Source: three-view drawing plus pictorial views. Frame: mm from the lowest corner of the part. A direction names the side the tool comes from. Coordinates: 2 decimals unless noted, no trailing zeros. Write each loop counter-clockwise with the first axis right and the second up, starting at its lowest first coordinate (ties: lowest second). Pieces come first, ordered by that corner, then holes. Notation, with made-up numbers: (67, 9) - (75, 9) arc R37 ccw to (75, 45) - close; hole circle Ø6 at (-18.5, 35.25). An arc over 180 degrees is marked (long way). Answer as a JSON object with one key per item and string values. Group by question number.
Item 1: Set-up query: the marked faces 1, 2 and 3. Return all of +Z, -Z, +X, -X, +Y, -Y with unobstructed straight access to the full face (end or side cutting, diameter ignored); none if empty.
Item 2: Section A-A on y = 5. Return loops of the section in (x, z).
Item 3: Section D-D on z = 2.5. Return loops of the section in (x, y), and give its area (3 significant figures).
Item 4: Mould query, pull axis Z, two halves, no side actions, for the marked faces 4, 5, 6 and 7. Classes: pulls with the +Z half, pulls with the -Z half, needs draft (parallel to the pull), parting line crosses it, or undercut.
Item 5: Section C-C on x = 8.5. Return loops of the section in (y, z).
Item 6: Section B-B on x = 5.5. Return loops of the section in (y, z).
Item 7: Line query: line 1 along Y through (x, z) = (7, 3); line 2 along X through (y, z) = (6.25, 6.5); line 3 along X through (y, z) = (1.75, 5.5). Output: solid intervals per line, ascending. Write a range as from..to.
Item 8: First-contact query: pin 1 Ø1 at (x, y) = (2.5, 4.5) entering from -Z; pin 2 Ø1.1 at (y, z) = (5, 6.5) entering from +X; pin 3 Ø0.8 at (x, y) = (9.5, 4) entering from -Z. Flat tips, straight axial feed; report the tip coordinate or a pass-through.
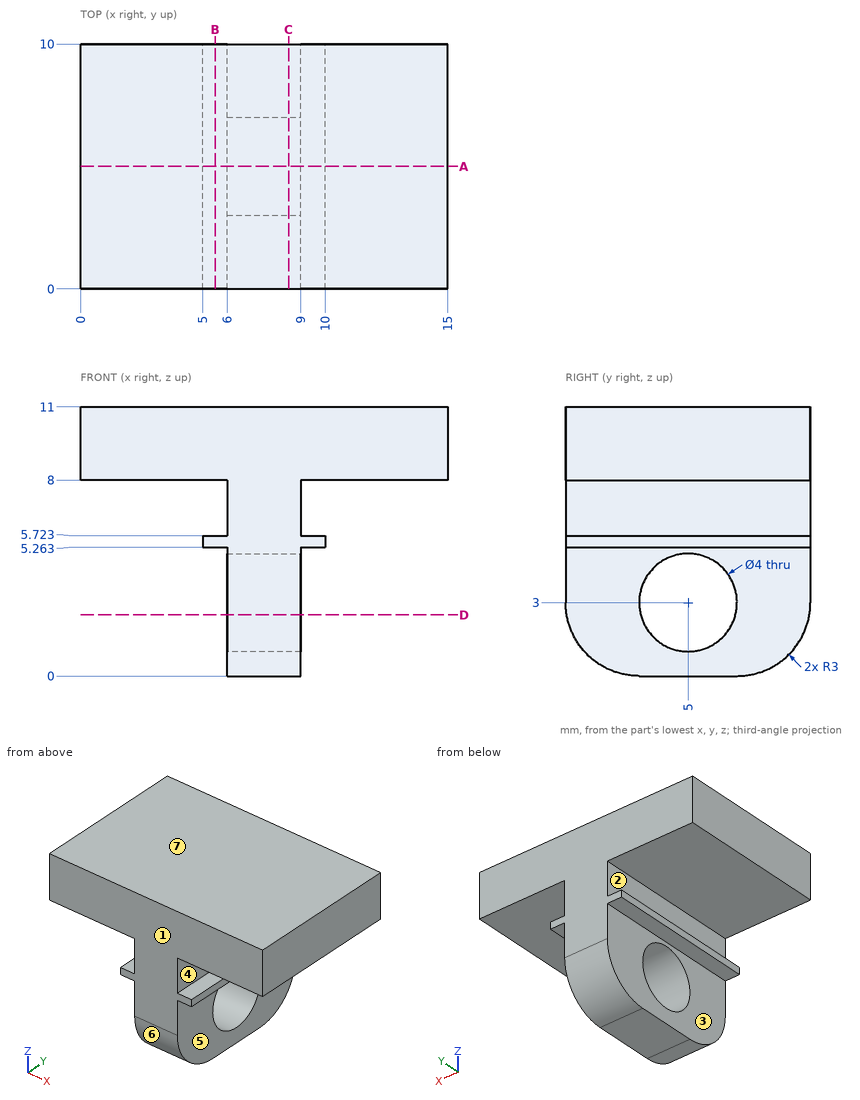
Checks:
{
 "1": {"face 1": "+Z, -Z, +X, -X, -Y", "face 2": "-X, +Y, -Y", "face 3": "-Z, -X, +Y, -Y"},
 "2": {"outline": "(0, 8) - (6, 8) - (6, 5.72) - (5, 5.72) - (5, 5.26) - (6, 5.26) - (6, 5) - (9, 5) - (9, 5.26) - (10, 5.26) - (10, 5.72) - (9, 5.72) - (9, 8) - (15, 8) - (15, 11) - (0, 11) - close; (6, 0) - (9, 0) - (9, 1) - (6, 1) - close"},
 "3": {"outline": "(6, 0.04) - (9, 0.04) - (9, 3.06) - (6, 3.06) - close; (6, 6.94) - (9, 6.94) - (9, 9.96) - (6, 9.96) - close", "area": "18.1 mm^2"},
 "4": {"face 4": "undercut", "face 5": "needs draft", "face 6": "pulls with the -Z half", "face 7": "pulls with the +Z half"},
 "5": {"outline": "(0, 3) arc R3 ccw to (3, 0) - (7, 0) arc R3 ccw to (10, 3) - (10, 11) - (0, 11) - close; hole circle Ø4 at (5, 3)"},
 "6": {"outline": "(0, 5.26) - (10, 5.26) - (10, 5.72) - (0, 5.72) - close; (0, 8) - (10, 8) - (10, 11) - (0, 11) - close"},
 "7": {"line 1": "0..3, 7..10", "line 2": "6..9", "line 3": "5..10"},
 "8": {"pin 1": "z = 8", "pin 2": "x = 9", "pin 3": "z = 5.26"}
}
